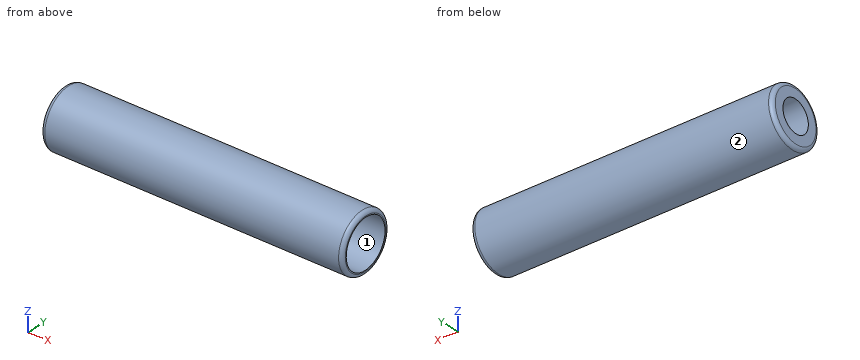
from build123d import *

# Parameters (mm, degrees)
ESBO_O1_W                  = 80
ESBO_O1_H                  = 7.8
ESBO_O2_R                  = 6.5
CORTE_EXTRUS_O1_DEPTH      = 25
CORTE_EXTRUS_O2_DEPTH      = 57.095276093
CORTE_EXTRUS_O2_DEPTH_BACK = 57.095276093
ESBO_O3_R                  = 4.25
FILETE1_R                  = 1


with BuildPart() as part:
    # Esboço1 → Revolução1 (revolve)
    with BuildSketch(Plane.XY, mode=Mode.PRIVATE) as revolu_o1_sk:
        with Locations((0, 3.9)):
            Rectangle(ESBO_O1_W, ESBO_O1_H)
    revolve(revolu_o1_sk.sketch.rotate(Axis((-40, 0, 0), (1, 0, 0)), 90), axis=Axis((-40, 0, 0), (1, 0, 0)))

    # Esboço2 → Corte-extrusão1 (cut)
    with BuildSketch(Plane(origin=(40, 0, 0), x_dir=(0, 0, -1), z_dir=(1, 0, 0))):
        Circle(ESBO_O2_R)
    extrude(amount=-CORTE_EXTRUS_O1_DEPTH, mode=Mode.SUBTRACT)

    # Esboço3 → Corte-extrusão2 (cut, two sides: drawn at the far end of the back side and taken through both)
    with BuildSketch(Plane(origin=(15, 0, 0), x_dir=(0, 0, -1), z_dir=(1, 0, 0)).offset(-CORTE_EXTRUS_O2_DEPTH_BACK)):
        Circle(ESBO_O3_R)
    extrude(amount=CORTE_EXTRUS_O2_DEPTH + CORTE_EXTRUS_O2_DEPTH_BACK, mode=Mode.SUBTRACT)

    # Filete1
    filete1_edges = [part.edges().sort_by_distance(p)[0] for p in [
        (-40, 0, -7.8),
        (40, 0, -7.8),
    ]]
    fillet(filete1_edges, radius=FILETE1_R)


solid = part.part
Geometry check sheet. Reference: the model listing, model coordinates, mm. Face numbers are marked on the shaded views. Give positions to 0.01 mm unless a question says otherwise; leave off trailing zeros. Order: outer loops, then holes, each group sorted by start corner. A loop starts at its lowest first (then second) coordinate and runs counter-clockwise, first axis right, second up. Notation, with made-up numbers: (-6.75, -34.75) - (19.25, -34.75) arc R26 cw to (19.25, -5.75) - close; hole circle Ø11 at (79.25, 13.5). An arc over 180 degrees is marked (long way). Answer as a JSON object with one key per item and string values.
(1) Cross-section at A-A (z = 0). Record the cut outline in (x, y), then the cut area to 3 significant figures.
Report:
{"outline": "(-40, -6.8) arc R1 ccw to (-39, -7.8) - (39, -7.8) arc R1 ccw to (40, -6.8) - (40, -6.5) - (15, -6.5) - (15, -4.25) - (-40, -4.25) - close; (-40, 4.25) - (15, 4.25) - (15, 6.5) - (40, 6.5) - (40, 6.8) arc R1 ccw to (39, 7.8) - (-39, 7.8) arc R1 ccw to (-40, 6.8) - close", "area": "455 mm^2"}
(2) Depth check by flat-ended pin: pin 1 Ø1.5 at (x, z) = (6.5, -4.5) entering from +Y; pin 2 Ø1.5 at (x, y) = (-21, -3) entering from +Z; pin 3 Ø2 at (x, y) = (1.5, 3.5) entering from +Z. Enter the tip coordinate at first touch or a pass-through.
Report:
{"pin 1": "y = 6.84", "pin 2": "z = 7.47", "pin 3": "z = 7.39"}
(3) Draft check along Z on the marked faces 1 and 2. Enter one of: released by +Z, released by -Z, zero draft, split by the parting line, or undercut.
Report:
{"face 1": "undercut", "face 2": "split by the parting line"}
(4) Material ranges on line 1 (Y direction, x = 22.5, z = 0); line 2 (X direction, y = -6, z = -0.75); line 3 (Y direction, x = -15.5, z = 0), recorded low to high.
Report:
{"line 1": "-7.8 to -6.5, 6.5 to 7.8", "line 2": "-40 to 15", "line 3": "-7.8 to -4.25, 4.25 to 7.8"}
(5) Cross-section at C-C (x = -23). Record the cut outline in (y, z).
Report:
{"outline": "circle Ø15.6 at (0, 0); hole circle Ø8.5 at (0, 0)"}
